Source: three-view drawing plus pictorial views. Frame: mm from the lowest corner of the part. A direction names the side the tool comes from. Round coordinates to 2 decimals unless told otherwise and drop trailing zeros. Loops run counter-clockwise (first coordinate to the right, second up) from the corner with the lowest first, then second, coordinate; pieces in that order, holes last. Notation, with made-up numbers: (59.25, 57.25) -> (110.25, 57.25) arc R17 cw to (110.25, 88.25) -> close; hole circle Ø6 at (79, 37). An arc over 180 degrees is marked (long way). Put each result on its own line as item: value. Start each with the question number.
1. Cut plane C-C (x = 17). Return the cut outline in (y, z), then the cut area to 3 significant figures.
2. Material intervals for L1, parallel to Y at x = 3.25, z = 21.25; L2, parallel to X at y = 15, z = 21; L3, parallel to Y at x = 52, z = 20 (1 decimal), sorted ascending.
3. Set-up query: the marked faces 4, 5, 6, 7 and 8. Return all of +Z, -Z, +X, -X, +Y, -Y with unobstructed straight access to the full face (end or side cutting, diameter ignored); none if empty.
4. Cut plane D-D (z = 8). Return the cut outline in (x, y).
5. Cut plane B-B (x = 52.75). Return the cut outline in (y, z).
6. Cut plane A-A (y = 18). Return the cut outline in (x, z).
7. Draft query along X for the marked faces 1, 2 and 3. Return one class per face: pulls with the +X half, pulls with the -X half, needs draft (parallel to the pull), parting line crosses it, or undercut.
8. Contact query for flat-ended pins moving along their axis: pin 1 (2.5 mm diameter, centred on x = 3, y = 4.5, fed in from -Z); pin 2 (8 mm diameter, centred on y = 6.5, z = 20.5, fed in from -X); pin 3 (12 mm diameter, centred on x = 41.5, y = 6, fed in from +Z); pin 4 (5.5 mm diameter, centred on x = 23, z = 28, fed in from -Y). Output: stop coordinate, or through.
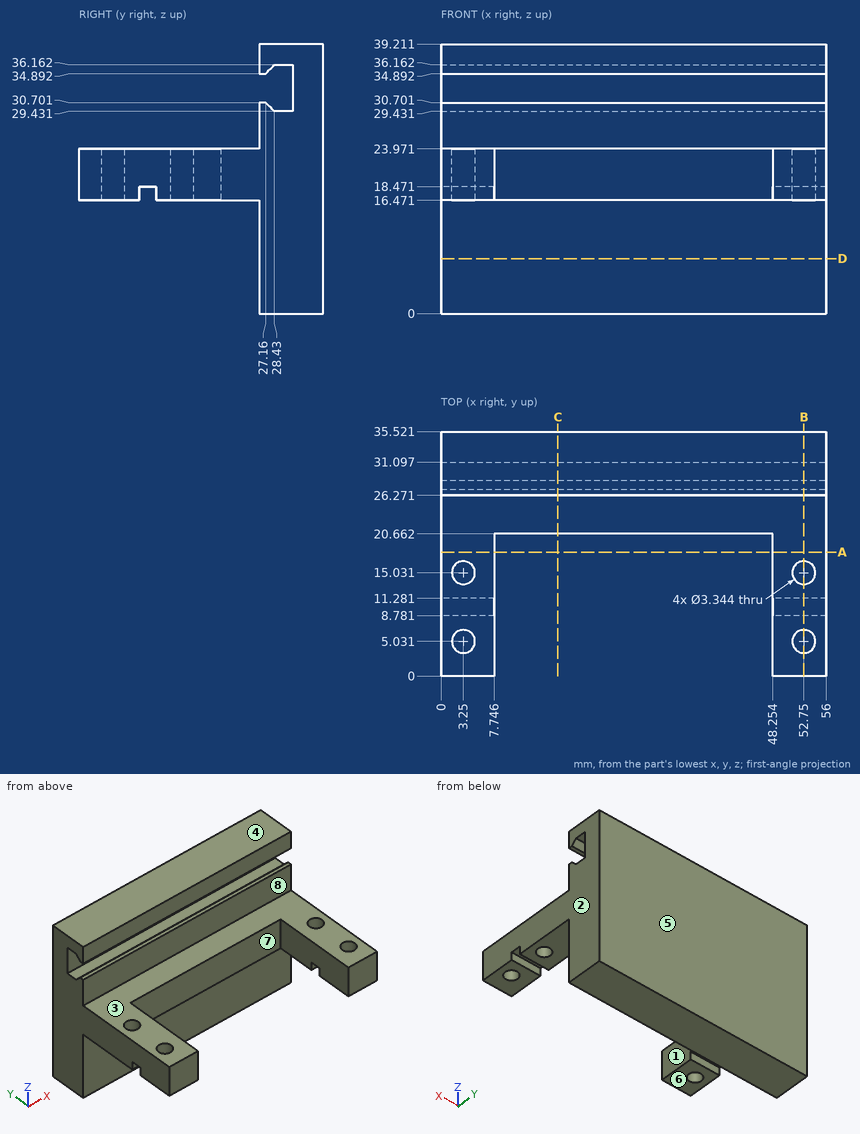
Solution:
1. outline: (20.66, 16.47) -> (26.27, 16.47) -> (26.27, 0) -> (35.52, 0) -> (35.52, 39.21) -> (26.27, 39.21) -> (26.27, 34.89) -> (27.16, 34.89) -> (28.43, 36.16) -> (31.1, 36.16) -> (31.1, 29.43) -> (28.43, 29.43) -> (27.16, 30.7) -> (26.27, 30.7) -> (26.27, 23.97) -> (20.66, 23.97) -> close
1. area: 376 mm^2
2. L1: y = 0 to 3.36, 6.7 to 13.36, 16.7 to 35.52
2. L2: x = 0 to 1.58, 4.92 to 7.75, 48.25 to 51.08, 54.42 to 56
2. L3: y = 0 to 3.5, 6.5 to 13.5, 16.5 to 35.5
3. face 4: +Z, +X, -X, +Y, -Y
3. face 5: +Z, -Z, +X, -X, +Y
3. face 6: -Z, +X, -X, -Y
3. face 7: +Z, -Z, -Y
3. face 8: +Z, +X, -X, -Y
4. outline: (0, 26.27) -> (56, 26.27) -> (56, 35.52) -> (0, 35.52) -> close
5. outline: (0, 16.47) -> (3.36, 16.47) -> (3.36, 23.97) -> (0, 23.97) -> close; (6.7, 16.47) -> (8.78, 16.47) -> (8.78, 18.47) -> (11.28, 18.47) -> (11.28, 16.47) -> (13.36, 16.47) -> (13.36, 23.97) -> (6.7, 23.97) -> close; (16.7, 16.47) -> (26.27, 16.47) -> (26.27, 0) -> (35.52, 0) -> (35.52, 39.21) -> (26.27, 39.21) -> (26.27, 34.89) -> (27.16, 34.89) -> (28.43, 36.16) -> (31.1, 36.16) -> (31.1, 29.43) -> (28.43, 29.43) -> (27.16, 30.7) -> (26.27, 30.7) -> (26.27, 23.97) -> (16.7, 23.97) -> close
6. outline: (0, 16.47) -> (7.75, 16.47) -> (7.75, 23.97) -> (0, 23.97) -> close; (48.25, 16.47) -> (56, 16.47) -> (56, 23.97) -> (48.25, 23.97) -> close
7. face 1: undercut
7. face 2: pulls with the +X half
7. face 3: needs draft
8. pin 1: stops at z = 16.47
8. pin 2: stops at x = 0
8. pin 3: passes through
8. pin 4: stops at y = 26.27
